Read the model definition and answer for the solid it produces. Units are mm, in the model's axes. Face numbers are marked on the shaded views. Round coordinates to 2 decimals unless told otherwise and drop trailing zeros. One line per item, written item: value. Start each with the question number.
1. The mould has two halves that part along Z. Classify the marked faces 1, 2, 3 and 4: released by +Z, released by -Z, zero draft, split by the parting line, or undercut.
2. Flat-ended cylindrical pins translate along their axes: pin 1 Ø0.7 at (x, z) = (-7.5, 24.5) entering from +Y; pin 2 Ø0.9 at (x, z) = (1.5, 27) entering from +Y; pin 3 Ø8 at (y, z) = (5.5, 2) entering from +X. Find the tip coordinate at first contact, or state that the pin passes through.
3. Consider line 1 (X direction, y = 4.9, z = -13); line 2 (X direction, y = 4.4, z = 3); line 3 (Y direction, x = 4, z = 0). Determine where each line is inside the solid, lowest interval first.
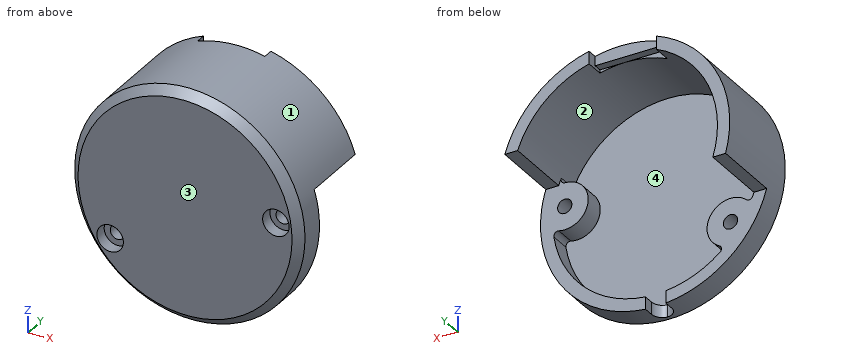
from build123d import *

# Parameters (mm, degrees)
SKETCH1_R           = 28.25
BOSS_EXTRUDE1_DEPTH = 25
SHELL1_T            = -3
CUT_EXTRUDE1_DEPTH  = 17
SKETCH3_W           = 16.5
SKETCH3_H           = 5.174038482
CUT_EXTRUDE2_DEPTH  = 2.5
CUT_EXTRUDE3_DEPTH  = 48.128812843
SKETCH6_R           = 3.25
CUT_EXTRUDE4_DEPTH  = 46.608387559
SKETCH7_R           = 5.75
SKETCH7_R_2         = 1.75
BOSS_EXTRUDE2_DEPTH = 5
FILLET1_R           = 1
CHAMFER1_SIZE       = 2
SKETCH8_W           = 16.5
SKETCH8_H           = 2.174038482
CUT_EXTRUDE5_DEPTH  = 2


with BuildPart() as part:
    # Sketch1 → Boss-Extrude1 (new body)
    with BuildSketch(Plane(origin=(0, 0, 0), x_dir=(1, 0, 0), z_dir=(0, 1, 0))):
        with Locations(Location((0, 0, 0), (0, 0, 270))):
            Circle(SKETCH1_R)
    extrude(amount=BOSS_EXTRUDE1_DEPTH)

    # Shell1
    shell1_openings = [part.faces().sort_by_distance(p)[0] for p in [
        (0, 25, 0),
    ]]
    offset(amount=SHELL1_T, openings=shell1_openings, kind=Kind.INTERSECTION)

    # Sketch2 → Cut-Extrude1 (cut)
    with BuildSketch(Plane(origin=(0, 25, 0), x_dir=(1, 0, 0), z_dir=(0, 1, 0))):
        Polygon((0, 7.5), (-28.25, 7.5), (-28.25, 28.25), (28.25, 28.25), (28.25, -8.5), (0, -8.5), align=None)
    extrude(amount=-CUT_EXTRUDE1_DEPTH, mode=Mode.SUBTRACT)

    # Sketch3 → Cut-Extrude2 (cut)
    with BuildSketch(Plane(origin=(0, 25, 0), x_dir=(1, 0, 0), z_dir=(0, 1, 0))):
        with Locations((-2, -25.662980759)):
            Rectangle(SKETCH3_W, SKETCH3_H)
    extrude(amount=-CUT_EXTRUDE2_DEPTH, mode=Mode.SUBTRACT)

    # Sketch5 → Cut-Extrude3 (cut, through all)
    with BuildSketch(Plane.XY):
        with BuildLine():
            Line((2.5, 8), (2.5, 5.5))
            ThreePointArc((2.5, 5.5), (1.767766953, 3.732233047), (0, 3))
            ThreePointArc((0, 3), (-1.767766953, 3.732233047), (-2.5, 5.5))
            Line((-2.5, 5.5), (-2.5, 8))
            Line((-2.5, 8), (2.5, 8))
        make_face()
    extrude(amount=-CUT_EXTRUDE3_DEPTH, mode=Mode.SUBTRACT)

    # Sketch6 → Cut-Extrude4 (cut, through all)
    with BuildSketch(Plane(origin=(0, 3, 0), x_dir=(1, 0, 0), z_dir=(0, 1, 0))):
        with Locations(Location((-18.364367672, 13, 0), (0, 0, 270))):
            Circle(SKETCH6_R)
        with Locations(Location((22.299103121, -3, 0), (0, 0, 270))):
            Circle(SKETCH6_R)
    extrude(amount=-CUT_EXTRUDE4_DEPTH, mode=Mode.SUBTRACT)

    # Sketch7 → Boss-Extrude2 (add)
    # profile 1 of 2: a face of its own
    with BuildSketch(Plane(origin=(0, 3, 0), x_dir=(1, 0, 0), z_dir=(0, 1, 0))):
        with Locations((-18.364367672, 13)):
            Circle(SKETCH7_R)
        with Locations(Location((-18.364367672, 13, 0), (0, 0, 90))):
            Circle(SKETCH7_R_2, mode=Mode.SUBTRACT)
    # profile 2 of 2: a face of its own
    with BuildSketch(Plane(origin=(0, 3, 0), x_dir=(1, 0, 0), z_dir=(0, 1, 0))):
        with Locations((22.299103121, -3)):
            Circle(SKETCH7_R)
        with Locations(Location((22.299103121, -3, 0), (0, 0, 90))):
            Circle(SKETCH7_R_2, mode=Mode.SUBTRACT)
    extrude(amount=BOSS_EXTRUDE2_DEPTH)

    # Fillet1
    fillet1_edges = [part.edges().sort_by_distance(p)[0] for p in [
        (-23.219797584, 5.5, -9.919853839),
        (-17.072985413, 5.5, -18.603109124),
        (23.753694458, 5.5, 8.56297259),
        (25.172189575, 5.5, -1.980750368),
    ]]
    fillet(fillet1_edges, radius=FILLET1_R)

    # Chamfer1
    chamfer1_edges = [part.edges().sort_by_distance(p)[0] for p in [
        (0, 0, -28.25),
    ]]
    chamfer(chamfer1_edges, length=CHAMFER1_SIZE)

    # Sketch8 → Cut-Extrude5 (cut)
    with BuildSketch(Plane(origin=(0, 22.5, 0), x_dir=(1, 0, 0), z_dir=(0, 1, 0))):
        with Locations((-2, -24.162980759)):
            Rectangle(SKETCH8_W, SKETCH8_H)
    extrude(amount=-CUT_EXTRUDE5_DEPTH, mode=Mode.SUBTRACT)


solid = part.part
Answer:
1. face 1: split by the parting line
1. face 2: undercut
1. face 3: zero draft
1. face 4: undercut
2. pin 1: y = 20.5
2. pin 2: y = 22.5
2. pin 3: x = 28.25
3. line 1: -25.08 to -20.11, -16.61 to -12.61, 21.65 to 25.08
3. line 2: -28.09 to -25.07, 16.55 to 20.55, 24.05 to 28.09
3. line 3: 0 to 3
